Geometry check sheet. Reference: the model listing, model coordinates, mm. A direction names the side the tool comes from. Give positions to 0.01 mm unless a question says otherwise; leave off trailing zeros. Write each loop counter-clockwise with the first axis right and the second up, starting at its lowest first coordinate (ties: lowest second). Pieces come first, ordered by that corner, then holes. Notation, with made-up numbers: (52, 78) - (92, 78) arc R14 cw to (92, 98) - close; hole circle Ø2 at (-28.75, 44.5). An arc over 180 degrees is marked (long way). Use a Markdown table: item, result.
Autodesk Inventor part; units mm, degrees
ref_plane "YZ Plane" through (0, 0, 0) normal (1, 0, 0) x (0, 1, 0)
ref_plane "XZ Plane" through (0, 0, 0) normal (0, 1, 0) x (-1, 0, 0)
ref_plane "XY Plane" through (0, 0, 0) normal (0, 0, 1) x (1, 0, 0)
sketch "Эскиз1" plane through (0, 0, 0) normal (0, 0, 1) x (1, 0, 0)
  line L0 (1, 0.1) -> (0, 1.1)
  line L1 (0, 1.1) -> (0, 3.35)
  line L2 (0, 3.35) -> (1.7, 4.1)
  line L3 (1.7, 4.1) -> (8, 4.1)
  line L4 (8, 4.1) -> (8, 4.85)
  line L5 (8, 4.85) -> (13, 4.85)
  line L6 (13, 4.85) -> (13, 3.65)
  line L7 (13, 3.65) -> (6, 0.1)
  line L8 (6, 0.1) -> (1, 0.1)
  line L9 (-2.6, 0) -> (15.6, 0) construction
  line L10 (0, -0.97) -> (0, 5.82) construction
  point P0 (0, 0)
  point P1 (0, -0.97)
  dimension "d1" = 0.1
  dimension "d2" = 4.1
  dimension "d3" = 1.7
  dimension "d5" = 3.35
  dimension "d6" = 1
  dimension "d7" = 135
  dimension "d8" = 5
  dimension "d9" = 13
  dimension "d10" = 4.85
  dimension "d11" = 5
  dimension "d12" = 1.2
revolve "Вращение1" add sketch "Эскиз1" angle 360 about axis through (-10, 0, 0) along (1, 0, 0)
properties part number "Сопло фильеры"
1) Section check B-B on x = 8.5. Record the boundary of the cut face in (y, z).
Working result:
| item | result |
|---|---|
| outline | circle Ø9.7 at (0, 0); hole circle Ø2.74 at (0, 0) |
2) Depth check by flat-ended pin: P1, Ø1, axis at x = 7, z = 1.5, coming from the -Y side; P2, Ø1, axis at x = 8.5, z = 3.5, coming from the -Y side; P3, Ø3, axis at x = 8, z = -3, coming from the -Y side. Enter the tip coordinate at first touch or a pass-through.
Working result:
| item | result |
|---|---|
| P1 | stops at y = -3.98 |
| P2 | stops at y = -3.81 |
| P3 | stops at y = -4.61 |
3) Material ranges on L1, parallel to Z at x = 4.85, y = 0; L2, parallel to X at y = 4.25, z = -1; L3, parallel to Y at x = 9.25, z = 0.75, recorded low to high. Write a range as from..to.
Working result:
| item | result |
|---|---|
| L1 | z = -4.1..-0.1, 0.1..4.1 |
| L2 | x = 8..13 |
| L3 | y = -4.79..-1.58, 1.58..4.79 |
4) Mould release check, pull along Y, two halves, no side actions. Record for faces 1 (the cylindrical face through (4.894, -0.534, 4.065)), 2 (the conical face through (0.83, 0.26, -0.08)), 3 (the flat face through (13, 1, 4)): pulls with the +Y half, pulls with the -Y half, needs draft (parallel to the pull), parting line crosses it, or undercut.
Working result:
| item | result |
|---|---|
| face 1 | parting line crosses it |
| face 2 | undercut |
| face 3 | needs draft |
5) Section check A-A on x = 4.5. Record the boundary of the cut face in (y, z), then the cut area to 3 significant figures.
Working result:
| item | result |
|---|---|
| outline | circle Ø8.2 at (0, 0); hole circle Ø0.2 at (0, 0) |
| area | 52.8 mm² |
6) Set-up check for faces 4 (the cylindrical face through (10.535, 4.626, 1.457)), 5 (the flat face through (8, -2, 4)): record each of +Z, -Z, +X, -X, +Y, -Y from which the full face is reachable in a straight line by a thin tool's end or side.
Working result:
| item | result |
|---|---|
| face 4 | +X, -X |
| face 5 | -X |
